The listing builds one solid part. Answer for the finished solid, in the listing's coordinates (mm). Face numbers are marked on the shaded views. A direction names the side the tool comes from. Give positions to 0.01 mm unless a question says otherwise; leave off trailing zeros. Order: outer loops, then holes, each group sorted by start corner. A loop starts at its lowest first (then second) coordinate and runs counter-clockwise, first axis right, second up. Notation, with made-up numbers: (-26, 1) - (19, 1) arc R20 ccw to (19, 20) - close; hole circle Ø5 at (5, -13). An arc over 180 degrees is marked (long way). Answer in a Markdown table with one row per item.
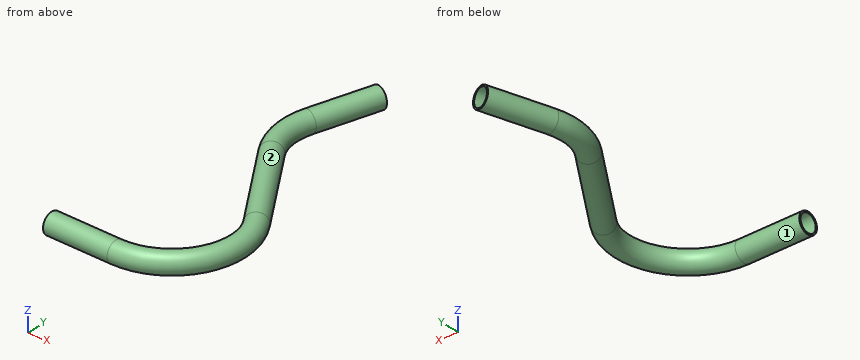
from build123d import *

# Parameters (mm, degrees)
ESQUISSE2_R   = 13.5
ESQUISSE2_R_2 = 11.5


with BuildPart() as part:
    # Balayage1: sweep along a path in Esquisse1
    with BuildLine(Plane.XY) as balayage1_path:
        Line((0, 0), (85, 0))
        ThreePointArc((85, 0), (160.39592082, 45.751367875), (154.627923765, 133.75399709))
        Line((154.627923765, 133.75399709), (74.327222675, 248.43528329))
        ThreePointArc((74.327222675, 248.43528329), (60.246487434, 282.429185278), (61.851451205, 319.188899214))
        Line((61.851451205, 319.188899214), (83.851070039, 401.292594448))
    # Esquisse2 → Balayage1 (sweep)
    with BuildSketch(Plane(origin=(0, 0, 0), x_dir=(0, 0, -1), z_dir=(1, 0, 0))):
        Circle(ESQUISSE2_R)
        Circle(ESQUISSE2_R_2, mode=Mode.SUBTRACT)
    sweep(path=balayage1_path.line)


solid = part.part
Item 1: Each of these flat-tipped pins is pushed along its axis until it touches: P1, Ø14, axis at y = 0, z = 0, coming from the +X side; P2, Ø10, axis at x = 33.5, z = -10.5, coming from the -Y side; P3, Ø8, axis at x = 75.5, y = 331, coming from the -Z side. Where does it stop, or does it pass through?
Answer block:
| item | result |
|---|---|
| P1 | x = 145.15 |
| P2 | y = -12.33 |
| P3 | z = -12.03 |
Item 2: Which of the six approach directions +Z, -Z, +X, -X, +Y, -Y give full straight-line access (tool end or side, diameter ignored) to the marked faces 1 and 2?
Answer block:
| item | result |
|---|---|
| face 1 | -X |
| face 2 | none |
Item 3: Find section B-B on x = 147.5. Count the separate pieces of the cut face and the enclosed holes in it, then the cut area to 3 significant figures.
Answer block:
| item | result |
|---|---|
| separate pieces | 2 |
| enclosed holes | 2 |
| area | 523 mm² |
Item 4: Consider line 1 (Y direction, x = 136, z = -5.5); line 2 (Y direction, x = 31.5, z = 0); line 3 (X direction, y = 332, z = 6.25). Determine where each line is inside the solid, lowest interval first.
Answer block:
| item | result |
|---|---|
| line 1 | 2.1 to 4.73, 30.14 to 33.23, 138.86 to 142.75, 177.97 to 181.85 |
| line 2 | -13.5 to -11.5, 11.5 to 13.5 |
| line 3 | 52.9 to 55.29, 75.28 to 77.67 |
Item 5: Find section A-A on z = -4. Write down the section's boundary in (x, y).
Answer block:
| item | result |
|---|---|
| outline | (0, -12.89) - (85, -12.89) arc R97.89 ccw to (165.19, 141.15) - (84.89, 255.83) arc R72.11 cw to (74.31, 315.85) - (96.31, 397.96) - (94.27, 398.5) - (72.27, 316.4) arc R74.22 ccw to (83.16, 254.62) - (163.46, 139.94) arc R95.78 cw to (85, -10.78) - (0, -10.78) - close; (0, 10.78) - (85, 10.78) arc R74.22 ccw to (145.8, 127.57) - (65.5, 242.25) arc R95.78 cw to (51.44, 321.98) - (73.44, 404.08) - (71.4, 404.63) - (49.4, 322.53) arc R97.89 ccw to (63.77, 241.04) - (144.07, 126.36) arc R72.11 cw to (85, 12.89) - (0, 12.89) - close |
